from build123d import *

# Parameters (mm, degrees)
SKETCH1_R           = 2.032
BOSS_EXTRUDE1_DEPTH = 1.5875
BOSS_EXTRUDE2_START = -15.065248
SKETCH2_R           = 2.032
BOSS_EXTRUDE2_DEPTH = 15.573248


with BuildPart() as part:
    # Sketch1 → Boss-Extrude1 (new body)
    with BuildSketch(Plane.XY):
        with BuildLine():
            ThreePointArc((-2.642212666, 4.009343348), (-11.808186134, -0.175285856), (-2.392603437, -3.763181293))
            ThreePointArc((-2.392603437, -3.763181293), (0, -2.73669663), (2.392603437, -3.763181293))
            ThreePointArc((2.392603437, -3.763181293), (11.808186134, -0.175285856), (2.642212666, 4.009343348))
            ThreePointArc((2.642212666, 4.009343348), (0, 2.974875822), (-2.642212666, 4.009343348))
        make_face()
        with Locations((-6.35, 0)):
            Circle(SKETCH1_R, mode=Mode.SUBTRACT)
        with Locations((6.35, 0)):
            Circle(SKETCH1_R, mode=Mode.SUBTRACT)
    boss_extrude1 = extrude(amount=BOSS_EXTRUDE1_DEPTH)

    # Sketch2 → Boss-Extrude2 (add)
    with BuildSketch(Plane(origin=(0, 0, 0), x_dir=(-1, 0, 0), z_dir=(0, 0, -1)).offset(BOSS_EXTRUDE2_START)):
        with Locations((6.35, 0)):
            Circle(SKETCH2_R)
    boss_extrude2 = extrude(amount=BOSS_EXTRUDE2_DEPTH)

    # Mirror2: Boss-Extrude1 across plane
    add(boss_extrude1.mirror(Plane(origin=(0, 0, 7.278624), x_dir=(1, 0, 0), z_dir=(0, 0, -1))))

    # Mirror3: Boss-Extrude2 across plane
    add(boss_extrude2.mirror(Plane(origin=(0, 0, 0), x_dir=(0, 0, 1), z_dir=(1, 0, 0))))


solid = part.part
Geometry check sheet. Reference: the model listing, model coordinates, mm. A direction names the side the tool comes from. Give positions to 0.01 mm unless a question says otherwise; leave off trailing zeros. Loops run counter-clockwise (first coordinate to the right, second up) from the corner with the lowest first, then second, coordinate; pieces in that order, holes last. Notation, with made-up numbers: M -23,55.5 L 4,55.5 A20 cw 4,63.5 Z; hole C 47,11.25 d11. An arc over 180 degrees is marked long. Write each question's results on one line, items separated by ' | '.
1) Section check A-A, the plane x = 6.35. Record the boundary of the cut face in (y, z), plus the area to 3 significant figures.
Answers follow:
outline: M -5.46,0 L -2.03,0 L -2.03,-0.51 L 2.03,-0.51 L 2.03,0 L 5.46,0 L 5.46,1.59 L 2.03,1.59 L 2.03,12.97 L 5.46,12.97 L 5.46,14.56 L 2.03,14.56 L 2.03,15.07 L -2.03,15.07 L -2.03,14.56 L -5.46,14.56 L -5.46,12.97 L -2.03,12.97 L -2.03,1.59 L -5.46,1.59 Z | area: 85.1 mm2
2) Section check C-C, the plane y = -3.5. Record the boundary of the cut face in (x, z).
Answers follow:
outline: M -10.54,0 L -2.11,0 L -2.11,1.59 L -10.54,1.59 Z; M -10.54,12.97 L -2.11,12.97 L -2.11,14.56 L -10.54,14.56 Z; M 2.11,0 L 10.54,0 L 10.54,1.59 L 2.11,1.59 Z; M 2.11,12.97 L 10.54,12.97 L 10.54,14.56 L 2.11,14.56 Z
3) Section check D-D, the plane x = -2. Record the boundary of the cut face in (y, z), plus the area to 3 significant figures.
Answers follow:
outline: M -3.41,0 L 3.53,0 L 3.53,1.59 L -3.41,1.59 Z; M -3.41,12.97 L 3.53,12.97 L 3.53,14.56 L -3.41,14.56 Z | area: 22.0 mm2
4) Gauge pin test, flat ends, axial feed: pin 1 (4 mm diameter, centred on x = 7.5, y = 3, fed in from -Z); pin 2 (5.5 mm diameter, centred on x = 2, y = -2.5, fed in from -Z); pin 3 (1.5 mm diameter, centred on y = -1.5, z = 5.5, fed in from +X); pin 4 (3 mm diameter, centred on y = -4, z = 9, fed in from -X). Record the tip position at first contact, or that the pin passes through.
Answers follow:
pin 1: z = -0.51 | pin 2: z = 0 | pin 3: x = 8.24 | pin 4: through
5) Thickness scan on line 1 (Z direction, x = -6.5, y = 4.75); line 2 (X direction, y = 1.5, z = 8.5); line 3 (X direction, y = -3.5, z = 13.5). Record the ranges inside material, lowest first.
Answers follow:
line 1: 0 to 1.59, 12.97 to 14.56 | line 2: -7.72 to -4.98, 4.98 to 7.72 | line 3: -10.54 to -2.11, 2.11 to 10.54
6) Tool access check on faces 3 (the face through (-4.32, 0.09, 14.81)), 4 (the face through (4.32, 0.09, -0.25)), 5 (the face through (11.8, -0.35, 0.78)), 6 (the face through (-0.037, -2.737, 13.775)), 7 (the face through (-4.32, 0.09, 7.36)). Record the directions out of +Z, -Z, +X, -X, +Y, -Y that give a thin tool (end or side, any length) a straight path to the whole face; none if there is none.
Answers follow:
face 3: +Z | face 4: -Z | face 5: +Z, -Z | face 6: +Z, -Z, -Y | face 7: none
7) Release check for a two-part mould opening along X. For faces 1 (the face through (6, 0, -0.508)), 2 (the face through (0, 0, 12.97)) record: +X half, -X half, draft (parallel to the pull), parting line (faces both ways), or undercut.
Answers follow:
face 1: draft | face 2: undercut
